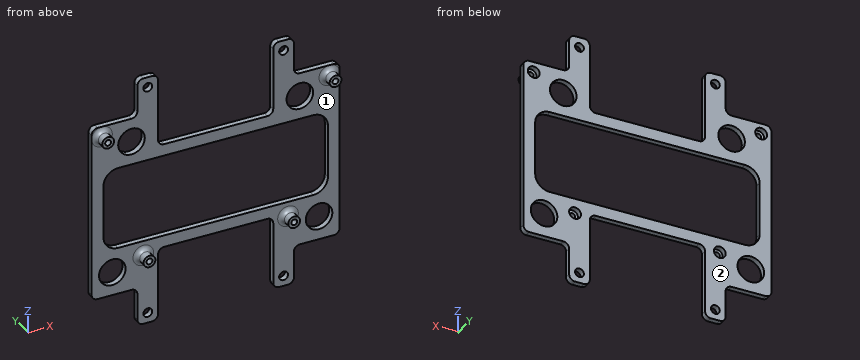
```python
from build123d import *

# Parameters (mm, degrees)
SKETCH_1_W          = 84
SKETCH_1_H          = 60
SKETCH_1_R          = 1
EXTRUDE_1_DEPTH     = 2
SKETCH_3_R          = 2
CUT_EXTRUDE_1_DEPTH = 1.9
SKETCH_4_R          = 2
SKETCH_4_R_2        = 1
EXTRUDE_2_DEPTH     = 4
FILLET_1_R          = 1.5
FILLET_3_R          = 2
SKETCH_6_W          = 7
SKETCH_6_H          = 13
SKETCH_6_R          = 1.5
EXTRUDE_4_DEPTH     = 2
CUT_EXTRUDE_2_REACH = 62.241
SKETCH_5_R          = 4.5
SKETCH_5_W          = 39
SKETCH_5_H          = 12
SKETCH_5_W_2        = 76
SKETCH_5_H_2        = 28
FILLET_6_R          = 2
FILLET_7_R          = 2
FILLET_8_R          = 5


with BuildPart() as part:
    # 草图1 → 凸台-拉伸1 (new body)
    with BuildSketch(Plane(origin=(0, 0, 0), x_dir=(1, 0, 0), z_dir=(0, 1, 0))):
        Rectangle(SKETCH_1_W, SKETCH_1_H)
        with Locations(Location((-38.5, -26.5, 0), (0, 0, 270))):
            Circle(SKETCH_1_R, mode=Mode.SUBTRACT)
        with Locations(Location((38.5, -26.5, 0), (0, 0, 270))):
            Circle(SKETCH_1_R, mode=Mode.SUBTRACT)
        with Locations(Location((-24.5, 19, 0), (0, 0, 270))):
            Circle(SKETCH_1_R, mode=Mode.SUBTRACT)
        with Locations(Location((24.5, 19, 0), (0, 0, 270))):
            Circle(SKETCH_1_R, mode=Mode.SUBTRACT)
    extrude(amount=EXTRUDE_1_DEPTH)

    # 草图3 → 切除-拉伸1 (cut)
    with BuildSketch(Plane(origin=(0, 2, 0), x_dir=(1, 0, 0), z_dir=(0, 1, 0))):
        with Locations(Location((-24.5, 19, 0), (0, 0, 270))):
            Circle(SKETCH_3_R)
        with Locations(Location((24.5, 19, 0), (0, 0, 270))):
            Circle(SKETCH_3_R)
        with Locations(Location((38.5, -26.5, 0), (0, 0, 270))):
            Circle(SKETCH_3_R)
        with Locations(Location((-38.5, -26.5, 0), (0, 0, 270))):
            Circle(SKETCH_3_R)
    extrude(amount=-CUT_EXTRUDE_1_DEPTH, mode=Mode.SUBTRACT)

    # 草图4 → 凸台-拉伸2 (add)
    # profile 1 of 4: a face of its own
    with BuildSketch(Plane.XZ):
        with Locations(Location((-38.5, 26.5, 0), (0, 0, 90))):
            Circle(SKETCH_4_R)
        with Locations(Location((-38.5, 26.5, 0), (0, 0, 270))):
            Circle(SKETCH_4_R_2, mode=Mode.SUBTRACT)
    # profile 2 of 4: a face of its own
    with BuildSketch(Plane.XZ):
        with Locations(Location((38.5, 26.5, 0), (0, 0, 90))):
            Circle(SKETCH_4_R)
        with Locations(Location((38.5, 26.5, 0), (0, 0, 270))):
            Circle(SKETCH_4_R_2, mode=Mode.SUBTRACT)
    # profile 3 of 4: a face of its own
    with BuildSketch(Plane.XZ):
        with Locations(Location((24.5, -19, 0), (0, 0, 90))):
            Circle(SKETCH_4_R)
        with Locations(Location((24.5, -19, 0), (0, 0, 270))):
            Circle(SKETCH_4_R_2, mode=Mode.SUBTRACT)
    # profile 4 of 4: a face of its own
    with BuildSketch(Plane.XZ):
        with Locations(Location((-24.5, -19, 0), (0, 0, 90))):
            Circle(SKETCH_4_R)
        with Locations(Location((-24.5, -19, 0), (0, 0, 270))):
            Circle(SKETCH_4_R_2, mode=Mode.SUBTRACT)
    extrude(amount=EXTRUDE_2_DEPTH)

    # 圆角1
    fillet_1_edges = [part.edges().sort_by_distance(p)[0] for p in [
        (-38.5, 0, 24.5),
        (38.5, 0, 24.5),
        (24.5, 0, -21),
        (-24.5, 0, -21),
    ]]
    fillet(fillet_1_edges, radius=FILLET_1_R - 0.0001)  # a hair under: the kernel refuses the full size

    # 圆角3
    fillet_3_edges = [part.edges().sort_by_distance(p)[0] for p in [
        (42, 1, 30),
        (-42, 1, 30),
        (-42, 1, -30),
        (42, 1, -30),
    ]]
    fillet(fillet_3_edges, radius=FILLET_3_R)

    # 草图6 → 凸台-拉伸4 (add)
    # profile 1 of 4: a face of its own
    with BuildSketch(Plane.XZ):
        with Locations((-23, 36.5)):
            Rectangle(SKETCH_6_W, SKETCH_6_H)
        with Locations(Location((-23, 39.5, 0), (0, 0, 270))):
            Circle(SKETCH_6_R, mode=Mode.SUBTRACT)
    # profile 2 of 4: a face of its own
    with BuildSketch(Plane.XZ):
        with Locations((23, 36.5)):
            Rectangle(SKETCH_6_W, SKETCH_6_H)
        with Locations(Location((23, 39.5, 0), (0, 0, 270))):
            Circle(SKETCH_6_R, mode=Mode.SUBTRACT)
    # profile 3 of 4: a face of its own
    with BuildSketch(Plane.XZ):
        with Locations((23, -36.5)):
            Rectangle(SKETCH_6_W, SKETCH_6_H)
        with Locations(Location((23, -39.5, 0), (0, 0, 270))):
            Circle(SKETCH_6_R, mode=Mode.SUBTRACT)
    # profile 4 of 4: a face of its own
    with BuildSketch(Plane.XZ):
        with Locations((-23, -36.5)):
            Rectangle(SKETCH_6_W, SKETCH_6_H)
        with Locations(Location((-23, -39.5, 0), (0, 0, 270))):
            Circle(SKETCH_6_R, mode=Mode.SUBTRACT)
    extrude(amount=-EXTRUDE_4_DEPTH)

    # 草图5 → 切除-拉伸2 (cut, up to next)
    with BuildSketch(Plane.XZ, mode=Mode.PRIVATE) as cut_extrude_2_sk1:
        with Locations(Location((-28.5, 22, 0), (0, 0, 270))):
            Circle(SKETCH_5_R)
    cut_extrude_2_tool1 = extrude(cut_extrude_2_sk1.sketch, amount=-CUT_EXTRUDE_2_REACH, mode=Mode.PRIVATE) & part.part
    # 草图5 → 切除-拉伸2 (cut, up to next)
    with BuildSketch(Plane.XZ, mode=Mode.PRIVATE) as cut_extrude_2_sk2:
        with Locations(Location((-35, -22, 0), (0, 0, 270))):
            Circle(SKETCH_5_R)
    cut_extrude_2_tool2 = extrude(cut_extrude_2_sk2.sketch, amount=-CUT_EXTRUDE_2_REACH, mode=Mode.PRIVATE) & part.part
    # 草图5 → 切除-拉伸2 (cut, up to next)
    with BuildSketch(Plane.XZ, mode=Mode.PRIVATE) as cut_extrude_2_sk3:
        with Locations(Location((35, -22, 0), (0, 0, 270))):
            Circle(SKETCH_5_R)
    cut_extrude_2_tool3 = extrude(cut_extrude_2_sk3.sketch, amount=-CUT_EXTRUDE_2_REACH, mode=Mode.PRIVATE) & part.part
    # 草图5 → 切除-拉伸2 (cut, up to next)
    with BuildSketch(Plane.XZ, mode=Mode.PRIVATE) as cut_extrude_2_sk4:
        with Locations(Location((28.5, 22, 0), (0, 0, 270))):
            Circle(SKETCH_5_R)
    cut_extrude_2_tool4 = extrude(cut_extrude_2_sk4.sketch, amount=-CUT_EXTRUDE_2_REACH, mode=Mode.PRIVATE) & part.part
    # 草图5 → 切除-拉伸2 (cut, up to next)
    with BuildSketch(Plane.XZ, mode=Mode.PRIVATE) as cut_extrude_2_sk5:
        with Locations((0, -24)):
            Rectangle(SKETCH_5_W, SKETCH_5_H)
    cut_extrude_2_tool5 = extrude(cut_extrude_2_sk5.sketch, amount=-CUT_EXTRUDE_2_REACH, mode=Mode.PRIVATE) & part.part
    # 草图5 → 切除-拉伸2 (cut, up to next)
    with BuildSketch(Plane.XZ, mode=Mode.PRIVATE) as cut_extrude_2_sk6:
        with Locations((0, 24)):
            Rectangle(SKETCH_5_W, SKETCH_5_H)
    cut_extrude_2_tool6 = extrude(cut_extrude_2_sk6.sketch, amount=-CUT_EXTRUDE_2_REACH, mode=Mode.PRIVATE) & part.part
    # 草图5 → 切除-拉伸2 (cut, up to next)
    with BuildSketch(Plane.XZ, mode=Mode.PRIVATE) as cut_extrude_2_sk7:
        Rectangle(SKETCH_5_W_2, SKETCH_5_H_2)
    cut_extrude_2_tool7 = extrude(cut_extrude_2_sk7.sketch, amount=-CUT_EXTRUDE_2_REACH, mode=Mode.PRIVATE) & part.part
    add(cut_extrude_2_tool1.solids().sort_by_distance((-28.5, 0, 22))[0], mode=Mode.SUBTRACT)
    add(cut_extrude_2_tool2.solids().sort_by_distance((-35, 0, -22))[0], mode=Mode.SUBTRACT)
    add(cut_extrude_2_tool3.solids().sort_by_distance((35, 0, -22))[0], mode=Mode.SUBTRACT)
    add(cut_extrude_2_tool4.solids().sort_by_distance((28.5, 0, 22))[0], mode=Mode.SUBTRACT)
    add(cut_extrude_2_tool5.solids().sort_by_distance((0, 0, -24))[0], mode=Mode.SUBTRACT)
    add(cut_extrude_2_tool6.solids().sort_by_distance((0, 0, 24))[0], mode=Mode.SUBTRACT)
    add(cut_extrude_2_tool7.solids().sort_by_distance((0, 0, 0))[0], mode=Mode.SUBTRACT)

    # 圆角6
    fillet_6_edges = [part.edges().sort_by_distance(p)[0] for p in [
        (-26.5, 1, 30),
        (26.5, 1, 30),
        (26.5, 1, -30),
        (-26.5, 1, -30),
        (19.5, 1, 18),
        (-19.5, 1, 18),
        (19.5, 1, -18),
        (-19.5, 1, -18),
    ]]
    fillet(fillet_6_edges, radius=FILLET_6_R)

    # 圆角7
    fillet_7_edges = [part.edges().sort_by_distance(p)[0] for p in [
        (-26.5, 1, 43),
        (-19.5, 1, 43),
        (19.5, 1, 43),
        (26.5, 1, 43),
        (19.5, 1, -43),
        (26.5, 1, -43),
        (-26.5, 1, -43),
        (-19.5, 1, -43),
    ]]
    fillet(fillet_7_edges, radius=FILLET_7_R)

    # 圆角8
    fillet_8_edges = [part.edges().sort_by_distance(p)[0] for p in [
        (-38, 1, 14),
        (-38, 1, -14),
        (38, 1, -14),
        (38, 1, 14),
    ]]
    fillet(fillet_8_edges, radius=FILLET_8_R)


solid = part.part
```
The listing builds one solid part. Answer for the finished solid, in the listing's coordinates (mm). Face numbers are marked on the shaded views. Round coordinates to 2 decimals unless told otherwise and drop trailing zeros. Loops run counter-clockwise (first coordinate to the right, second up) from the corner with the lowest first, then second, coordinate; pieces in that order, holes last.
Q1. For a pull along X with two mould halves and no side action, classify the marked faces 1 and 2 as released by +X, released by -X, zero draft, split by the parting line, or undercut.
Q2. Section C-C, the plane x = -2 is taken. Determine the outline of the cut face in (y, z).
Q3. Section B-B, the plane z = -7 is taken. Determine the outline of the cut face in (x, y).
Q4. Given pin 1 Ø2.5 at (x, z) = (23, -39.5) entering from +Y; pin 2 Ø1 at (y, z) = (1, -35) entering from -X; pin 3 Ø5 at (x, z) = (-23, -39.5) entering from -Y; pin 4 Ø2.5 at (x, z) = (-38.5, 26.5) entering from +Y, each flat-ended and moving along its own axis, determine where each tip first touches the part or whether it passes through.
Q5. Section D-D, the plane z = 39.5 is taken. Determine the outline of the cut face in (x, y), then the cut area to 3 significant figures.
Q6. Find the intervals of material crossed by line 1 (X direction, y = 0.75, z = 39.5); line 2 (X direction, y = -3.05, z = -19); line 3 (Z direction, x = -6.5, y = 0.3), in increasing order.
Q7. Section A-A, the plane y = -2.7 is taken. Determine the outline of the cut face in (x, z), then the cut area to 3 significant figures.
Completed:
1. face 1: undercut
1. face 2: zero draft
2. outline: (0, -18) - (2, -18) - (2, -14) - (0, -14) - close; (0, 14) - (2, 14) - (2, 18) - (0, 18) - close
3. outline: (-42, 0) - (-38, 0) - (-38, 2) - (-42, 2) - close; (38, 0) - (42, 0) - (42, 2) - (38, 2) - close
4. pin 1: passes through
4. pin 2: stops at x = -26.5
4. pin 3: stops at y = 0
4. pin 4: stops at y = 0.1
5. outline: (-26.5, 0) - (-24.5, 0) - (-24.5, 2) - (-26.5, 2) - close; (-21.5, 0) - (-19.5, 0) - (-19.5, 2) - (-21.5, 2) - close; (19.5, 0) - (21.5, 0) - (21.5, 2) - (19.5, 2) - close; (24.5, 0) - (26.5, 0) - (26.5, 2) - (24.5, 2) - close
5. area: 16.0 mm2
6. line 1: x = -26.5 to -24.5, -21.5 to -19.5, 19.5 to 21.5, 24.5 to 26.5
6. line 2: x = -26.5 to -25.5, -23.5 to -22.5, 22.5 to 23.5, 25.5 to 26.5
6. line 3: z = -18 to -14, 14 to 18
7. outline: circle Ø4 at (-38.5, 26.5); circle Ø4 at (-24.5, -19); circle Ø4 at (24.5, -19); circle Ø4 at (38.5, 26.5); hole circle Ø2 at (-38.5, 26.5); hole circle Ø2 at (-24.5, -19); hole circle Ø2 at (24.5, -19); hole circle Ø2 at (38.5, 26.5)
7. area: 37.7 mm2
